Geometry check sheet. Reference: the model listing, model coordinates, mm. Coordinates: 2 decimals unless noted, no trailing zeros. Order: outer loops, then holes, each group sorted by start corner. A loop starts at its lowest first (then second) coordinate and runs counter-clockwise, first axis right, second up. Notation, with made-up numbers: (14.25, -5) - (57.25, -5) arc R15 ccw to (57.25, 10) - close; hole circle Ø7 at (4, -39). An arc over 180 degrees is marked (long way). Put each result on its own line as item: value.
Autodesk Inventor part; units mm, degrees
ref_plane "YZ Plane" through (0, 0, 0) normal (1, 0, 0) x (0, 1, 0)
ref_plane "XZ Plane" through (0, 0, 0) normal (0, 1, 0) x (-1, 0, 0)
ref_plane "XY Plane" through (0, 0, 0) normal (0, 0, 1) x (1, 0, 0)
sketch "Sketch1" plane through (0, 0, 0) normal (0, 1, 0) x (-1, 0, 0)
  circle A0 centre (0, 0) radius 18
  circle A1 centre (0, 0) radius 22
  dimension "d0" = 36
  dimension "d1" = 44
extrude "Extrusion1" add sketch "Sketch1" along normal blind 30
sketch "Sketch2" plane through (0, 30, 0) normal (0, 1, 0) x (1, 0, 0)
  circle A0 centre (-20, 0) radius 1.175
  circle A1 centre (-17.3205, -10) radius 1.175
  circle A2 centre (-10, -17.3205) radius 1.175
  circle A3 centre (0, -20) radius 1.175
  circle A4 centre (10, -17.3205) radius 1.175
  circle A5 centre (17.3205, -10) radius 1.175
  circle A6 centre (20, 0) radius 1.175
  circle A7 centre (17.3205, 10) radius 1.175
  circle A8 centre (10, 17.3205) radius 1.175
  circle A9 centre (0, 20) radius 1.175
  circle A10 centre (-10, 17.3205) radius 1.175
  circle A11 centre (-17.3205, 10) radius 1.175
  point P0 (0, 0)
  dimension "d4" = 2.35
  dimension "d5" = 0
  dimension "d6" = 20
  dimension "d9" = 360
extrude "Extrusion2" cut sketch "Sketch2" against normal through all
properties part number "drive_sprocket_middle"
Q1. Section check A-A on x = 0. Record the boundary of the cut face in (y, z) (3 decimals), then the cut area to 3 significant figures.
Answer block:
outline: (0, -22) - (30, -22) - (30, -21.175) - (0, -21.175) - close; (0, -18.825) - (30, -18.825) - (30, -18) - (0, -18) - close; (0, 18) - (30, 18) - (30, 18.825) - (0, 18.825) - close; (0, 21.175) - (30, 21.175) - (30, 22) - (0, 22) - close
area: 99.0 mm^2
Q2. Draft check along X on faces 1 (the cylindrical face through (-0.153, 15.21, -21.165)), 2 (the cylindrical face through (4.769, 14.79, 21.477)), 3 (the flat face through (8.3, 30, 16.4)). Enter one of: pulls with the +X half, pulls with the -X half, needs draft (parallel to the pull), parting line crosses it, or undercut.
Answer block:
face 1: undercut
face 2: parting line crosses it
face 3: needs draft
Q3. Depth check by flat-ended pin: pin 1 Ø1.9 at (x, z) = (-10, 17.32) entering from -Y; pin 2 Ø6 at (y, z) = (15.5, 6.5) entering from -X; pin 3 Ø1 at (y, z) = (6.5, 11) entering from +X; pin 4 Ø1.5 at (y, z) = (18, -6.5) entering from +X. Enter the tip coordinate at first touch or a pass-through.
Answer block:
pin 1: passes through
pin 2: stops at x = -21.72
pin 3: stops at x = 19.33
pin 4: stops at x = 21.24
Q4. Thickness scan on L1, parallel to Z at x = 0, y = 23.5 (3 decimals); L2, parallel to X at y = 13.5, z = 0.5; L3, parallel to X at y = 5, z = -9.5. Record the ranges inside material, lowest first. Write a range as [from, to].
Answer block:
L1: z = [-22, -21.175], [-18.825, -18], [18, 18.825], [21.175, 22]
L2: x = [-21.99, -21.06], [-18.94, -17.99], [17.99, 18.94], [21.06, 21.99]
L3: x = [-19.84, -18.38], [-16.26, -15.29], [15.29, 16.26], [18.38, 19.84]
Q5. Section check C-C on y = 7.5. State how many separate pieces and enclosed holes the cut face has, then the cut area to 3 significant figures.
Answer block:
separate pieces: 1
enclosed holes: 13
area: 451 mm^2
Q6. Section check D-D on z = -10. Record the boundary of the cut face in (x, y).
Answer block:
outline: (-19.6, 0) - (-18.5, 0) - (-18.5, 30) - (-19.6, 30) - close; (-16.15, 0) - (-14.97, 0) - (-14.97, 30) - (-16.15, 30) - close; (14.97, 0) - (16.15, 0) - (16.15, 30) - (14.97, 30) - close; (18.5, 0) - (19.6, 0) - (19.6, 30) - (18.5, 30) - close
Q7. Section check B-B on z = 2.5. Record the boundary of the cut face in (x, y), then the cut area to 3 significant figures.
Answer block:
outline: (-21.86, 0) - (-17.83, 0) - (-17.83, 30) - (-21.86, 30) - close; (17.83, 0) - (21.86, 0) - (21.86, 30) - (17.83, 30) - close
area: 242 mm^2
